```python
from build123d import *

# Parameters (mm, degrees)
SALIENTE_EXTRUIR1_DEPTH = 310


with BuildPart() as part:
    # Croquis1 → Saliente-Extruir1 (new body)
    with BuildSketch(Plane(origin=(0, 0, 0), x_dir=(1, 0, 0), z_dir=(0, 1, 0))):
        with BuildLine():
            Line((4.625, 10), (0, 10))
            ThreePointArc((0, 10), (-1.414213562, 9.414213562), (-2, 8))
            Line((-2, 8), (-2, 2))
            ThreePointArc((-2, 2), (-1.414213562, 0.585786438), (0, 0))
            Line((0, 0), (16, 0))
            ThreePointArc((16, 0), (17.414213562, 0.585786438), (18, 2))
            Line((18, 2), (18, 8))
            ThreePointArc((18, 8), (17.41421361, 9.41421365), (16, 10.000000135))
            Line((16, 10.000000135), (11.374999664, 10.000000135))
            ThreePointArc((11.374999664, 10.000000135), (10.809314239, 9.76568556), (10.574999664, 9.200000135))
            Line((10.574999664, 9.200000135), (10.574999664, 8.500000898))
            ThreePointArc((10.574999664, 8.500000898), (10.662867611, 8.287868883), (10.87499961, 8.200000898))
            Line((10.87499961, 8.200000898), (13.044121001, 8.200000507))
            ThreePointArc((13.044121001, 8.200000507), (13.764747104, 7.718493399), (13.595664288, 6.868456885))
            Line((13.595664288, 6.868456885), (11.255887257, 4.528679854))
            ThreePointArc((11.255887257, 4.528679854), (10.282617211, 3.8783616), (9.134566914, 3.650000197))
            Line((9.134566914, 3.650000197), (6.865432698, 3.650000197))
            ThreePointArc((6.865432698, 3.650000197), (5.7173824, 3.878361599), (4.744112353, 4.528679854))
            Line((4.744112353, 4.528679854), (2.404335323, 6.868456883))
            ThreePointArc((2.404335323, 6.868456883), (2.23525255, 7.718493184), (2.955878471, 8.200000172))
            Line((2.955878471, 8.200000172), (5.124999858, 8.200000566))
            ThreePointArc((5.124999858, 8.200000566), (5.337131996, 8.287868609), (5.425, 8.500000763))
            Line((5.425, 8.500000763), (5.425, 9.2))
            ThreePointArc((5.425, 9.2), (5.190685425, 9.765685425), (4.625, 10))
        make_face()
    extrude(amount=SALIENTE_EXTRUIR1_DEPTH)


solid = part.part
```
Verification items for the finished model (mm, model axes). Coordinates: 2 decimals unless noted, no trailing zeros. Order: outer loops, then holes, each group sorted by start corner. A loop starts at its lowest first (then second) coordinate and runs counter-clockwise, first axis right, second up. Notation, with made-up numbers: (71, -2) - (107, -2) arc R10 cw to (107, 3) - close; hole circle Ø8 at (14, -8). An arc over 180 degrees is marked (long way). Return JSON: item names as keys, results as strings.
(1) Thickness scan on line 1 along X through (y, z) = (189.5, -8); line 2 along X through (y, z) = (230, -7.5); line 3 along Z through (x, y) = (7.25, 235.5). Record the ranges inside material, lowest first.
Filled sheet:
{"line 1": "x = -2 to 2.43, 13.57 to 18", "line 2": "x = -2 to 2.18, 13.82 to 18", "line 3": "z = -3.65 to 0"}
(2) Section check A-A, the plane y = 127. Record the cut outline in (x, z) (3 decimals), and give its area (3 significant figures).
Filled sheet:
{"outline": "(-2, -8) arc R2 ccw to (0, -10) - (4.625, -10) arc R0.8 ccw to (5.425, -9.2) - (5.425, -8.5) arc R0.3 ccw to (5.125, -8.2) - (2.956, -8.2) arc R0.78 cw to (2.404, -6.868) - (4.744, -4.529) arc R3 cw to (6.865, -3.65) - (9.135, -3.65) arc R3 cw to (11.256, -4.529) - (13.596, -6.868) arc R0.78 cw to (13.044, -8.2) - (10.875, -8.2) arc R0.3 ccw to (10.575, -8.5) - (10.575, -9.2) arc R0.8 ccw to (11.375, -10) - (16, -10) arc R2 ccw to (18, -8) - (18, -2) arc R2 ccw to (16, 0) - (0, 0) arc R2 ccw to (-2, -2) - close", "area": "147 mm^2"}
(3) Go/stop test with flat-tipped pins: pin 1 (1.5 mm diameter, centred on x = 10, z = -5, fed in from +Y); pin 2 (1.7 mm diameter, centred on x = 4.5, y = 185.5, fed in from +Z); pin 3 (2.5 mm diameter, centred on x = 7.5, y = 225, fed in from -Z); pin 4 (0.6 mm diameter, centred on y = 175.5, z = -9, fed in from +X). Record where each tip stops, or that it passes through.
Filled sheet:
{"pin 1": "passes through", "pin 2": "stops at z = 0", "pin 3": "stops at z = -3.71", "pin 4": "stops at x = 17.87"}
